from build123d import *

# Parameters (mm, degrees)
SKETCH2_R           = 49.53
BOSS_EXTRUDE1_DEPTH = 203.2
SKETCH3_R           = 12.411567775
BOSS_EXTRUDE2_DEPTH = 50.8
SKETCH4_R           = 49.53
CUT_EXTRUDE1_DEPTH  = 381
SHELL1_T            = -3.81


with BuildPart() as part:
    # Sketch1 → Revolve2 (revolve)
    with BuildSketch(Plane(origin=(0, 0, 0), x_dir=(1, 0, 0), z_dir=(0, 1, 0))):
        with BuildLine():
            Line((355.600000053, 50.799999973), (355.600000053, 1.269999973))
            Line((355.600000053, 1.269999973), (50.800000047, 1.269999973))
            Line((50.800000047, 1.269999973), (50.800000047, 13.68156774))
            add(Edge.make_bspline(
                [(50.800000047, 13.68156774), (51.224607869, 13.786541703), (52.079748124, 13.99736018), (53.901316113, 14.445024847), (55.90428978, 14.933081433), (57.918204029, 15.420277853), (59.969167456, 15.913068852), (62.005618607, 16.398707152), (64.04585603, 16.881716673), (66.619566178, 17.486536085), (69.727395203, 18.209576077), (73.370678613, 19.04644661), (77.55044141, 19.991710093), (82.779136229, 21.155661521), (97.433989811, 24.348822924), (119.485629173, 28.81699746), (168.00075752, 37.516041455), (219.035004801, 44.081341124), (262.822405655, 47.820230422), (299.206459448, 49.570692635), (308.841173655, 49.947366018), (315.265578413, 50.162354186), (319.548981494, 50.29122703), (323.832782669, 50.405645805), (328.116966628, 50.505609209), (332.401425999, 50.591116104), (336.139078075, 50.653092889), (339.329601827, 50.697064227), (341.973247658, 50.727612371), (344.069774299, 50.748376802), (346.163273231, 50.76568058), (348.272494467, 50.77952366), (350.344714481, 50.789906003), (352.405704949, 50.79682758), (354.282013928, 50.799423175), (355.162608625, 50.799999974), (355.600000053, 50.799999973)],
                knots=[0.08282658, 0.08282658, 0.08282658, 0.08282658, 0.08282658, 0.088510594, 0.094194608, 0.099878623, 0.105562637, 0.111246651, 0.116930666, 0.12261468, 0.128298694, 0.139917182, 0.15153567, 0.163154157, 0.174772645, 0.198009616, 0.314194483, 0.407142375, 0.709223026, 0.755696971, 0.790552431, 0.802170918, 0.813789405, 0.825407891, 0.837026378, 0.848644864, 0.860263351, 0.871881838, 0.877565852, 0.883249866, 0.88893388, 0.894617894, 0.900301908, 0.905985922, 0.911669936, 0.91735395, 0.91735395, 0.91735395, 0.91735395, 0.91735395], degree=4))
        make_face()
    revolve(axis=Axis((355.600000053, 0, -1.269999973), (-1, 0, 0)))

    # Sketch2 → Boss-Extrude1 (add)
    with BuildSketch(Plane(origin=(355.600000053, 0, 0), x_dir=(0, 0, -1), z_dir=(1, 0, 0))):
        with Locations((1.269999973, 0)):
            Circle(SKETCH2_R)
    extrude(amount=BOSS_EXTRUDE1_DEPTH)

    # Sketch3 → Boss-Extrude2 (add)
    with BuildSketch(Plane.ZY.offset(-50.800000063)):
        with Locations((-1.269999973, 0)):
            Circle(SKETCH3_R)
    extrude(amount=BOSS_EXTRUDE2_DEPTH)

    # Sketch4 → Cut-Extrude1 (cut)
    with BuildSketch(Plane(origin=(368.300000053, 0, 0), x_dir=(0, 0, -1), z_dir=(1, 0, 0))):
        with Locations((1.269999973, 0)):
            Circle(SKETCH4_R)
    extrude(amount=-CUT_EXTRUDE1_DEPTH, mode=Mode.SUBTRACT)

    # Shell1
    shell1_openings = [part.faces().sort_by_distance(p)[0] for p in [
        (558.800000053, 0, -1.269999973),
        (368.300000053, 0, -1.269999973),
    ]]
    offset(amount=SHELL1_T, openings=shell1_openings, kind=Kind.INTERSECTION)


solid = part.part
Verification items for the finished model (mm, model axes). Give positions to 0.01 mm unless a question says otherwise; leave off trailing zeros. Write each loop counter-clockwise with the first axis right and the second up, starting at its lowest first coordinate (ties: lowest second). Pieces come first, ordered by that corner, then holes.
(1) Gauge pin test, flat ends, axial feed: pin 1 (6 mm diameter, centred on x = 482, z = -31, fed in from -Y); pin 2 (2 mm diameter, centred on x = 445.5, z = -20, fed in from +Y); pin 3 (1 mm diameter, centred on x = 414, y = 37.5, fed in from -Z). Record the tip position at first contact, or that the pin passes through.
(2) Cross-section at A-A (z = -1.27). Enter the section's corners in (x, y), plus the area to 3 significant figures.
(3) Cross-section at B-B (y = 0). Enter the section's corners in (x, z).
(4) Material ranges on line 1 (Y direction, x = 467, z = -1.27); line 2 (Y direction, x = 547, z = -17.5); line 3 (Z direction, x = 403.5, y = 8), recorded low to high.
(5) Cross-section at C-C (x = 545.5). Enter the section's corners in (y, z).
(6) Mould release check, pull along Y, two halves, no side actions. Record for faces 1 (the face through (462.22, 13.73, -44.88)), 2 (the face through (462.22, 33.47, 35.24)), 3 (the face through (368.3, -44, -16)): +Y half, -Y half, draft (parallel to the pull), parting line (faces both ways), or undercut.
Worked out:
1. pin 1: stops at y = -41.7
1. pin 2: stops at y = 46.25
1. pin 3: stops at z = -34.2
2. outline: (368.3, -49.53) - (558.8, -49.53) - (558.8, -45.72) - (368.3, -45.72) - close; (368.3, 45.72) - (558.8, 45.72) - (558.8, 49.53) - (368.3, 49.53) - close
2. area: 1,450 mm2
3. outline: (368.3, -50.8) - (558.8, -50.8) - (558.8, -46.99) - (368.3, -46.99) - close; (368.3, 44.45) - (558.8, 44.45) - (558.8, 48.26) - (368.3, 48.26) - close
4. line 1: y = -49.53 to -45.72, 45.72 to 49.53
4. line 2: y = -46.8 to -42.74, 42.74 to 46.8
4. line 3: z = -50.15 to -46.28, 43.74 to 47.61
5. outline: circle Ø99.06 at (0, -1.27); hole circle Ø91.44 at (0, -1.27)
6. face 1: undercut
6. face 2: parting line
6. face 3: draft
